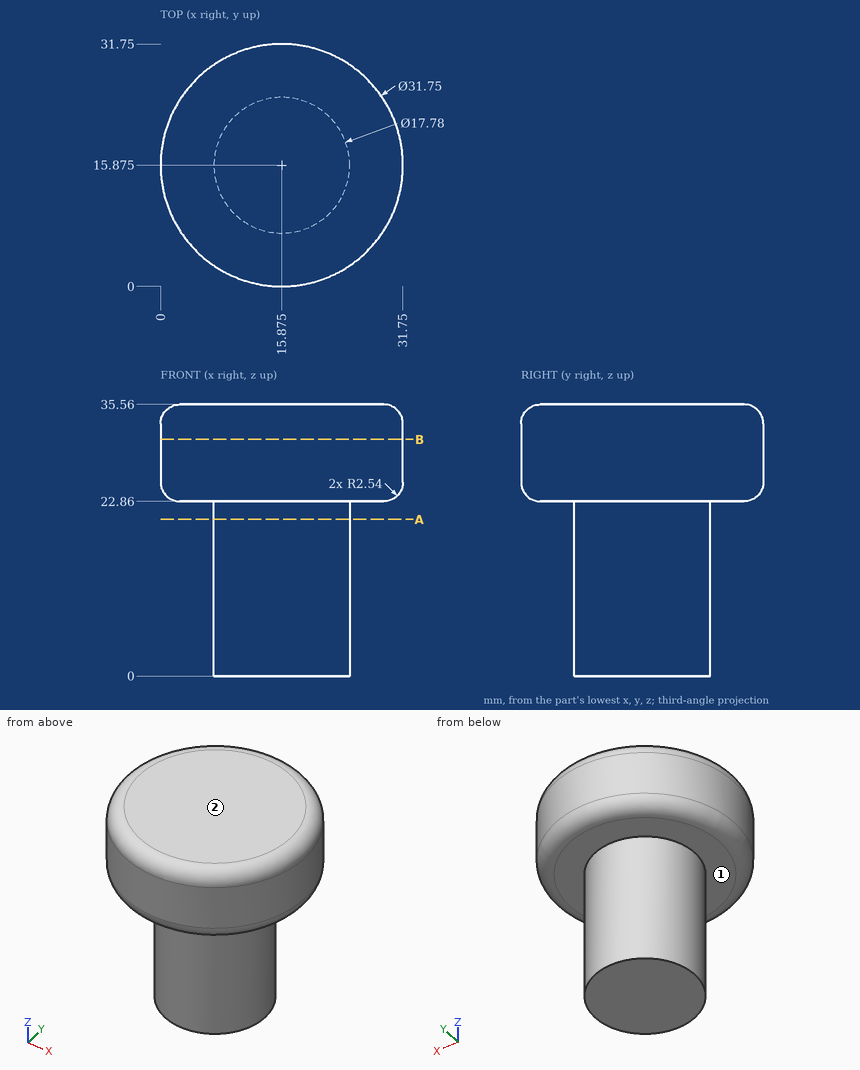
Answer from the drawing. Dimensions are ordinates in mm from the lowest x, y and z of the part. A direction names the side the tool comes from. Round coordinates to 2 decimals unless told otherwise and drop trailing zeros. Write each loop counter-clockwise with the first axis right and the second up, starting at its lowest first coordinate (ties: lowest second). Pieces come first, ordered by that corner, then holes. Notation, with made-up numbers: (61, -13.5) - (67, -13.5) arc R26 cw to (67, 11.5) - close; hole circle Ø10 at (1, -5.5). An arc over 180 degrees is marked (long way). One line per item, written item: value.
Q1. Find section A-A (z = 20.5). Determine the outline of the cut face in (x, y) (3 decimals).
The answers:
outline: circle Ø17.78 at (15.875, 15.875)
Q2. Straight lines are drawn through the part: line 1 (Y direction, x = 16, z = 14); line 2 (Y direction, x = 16, z = 29). For each, find the intervals that lie inside material, in ascending order. Write a range as from..to.
The answers:
line 1: y = 6.99..24.76
line 2: y = 0..31.75
Q3. Which of the six approach directions +Z, -Z, +X, -X, +Y, -Y give full straight-line access (tool end or side, diameter ignored) to the marked faces 1 and 2?
The answers:
face 1: -Z
face 2: +Z, +X, -X, +Y, -Y
Q4. Find section B-B (z = 31). Determine the outline of the cut face in (x, y) (3 decimals).
The answers:
outline: circle Ø31.75 at (15.875, 15.875)
Q5. Each of these flat-tipped pins is pushed along its axis until it touches: P1, Ø2, axis at x = 8.5, y = 21.5, coming from the -Z side; P2, Ø10, axis at x = 27.5, z = 13.5, coming from the +Y side; P3, Ø1, axis at x = 24, z = 9.5, coming from the -Y side; P4, Ø4, axis at y = 28, z = 28, coming from the +X side. Where does it stop, or does it pass through?
The answers:
P1: stops at z = 0
P2: stops at y = 21.8
P3: stops at y = 11.3
P4: stops at x = 28.1
